from build123d import *

# Parameters (mm, degrees)
F1_DEPTH = 20
F2_R     = 30
F3_T     = -2.5
F4_W     = 2.5
F4_H     = 2.5
F5_DEPTH = 15


with BuildPart() as f1:
    # F0 (on Top) → F1 (new body)
    with BuildSketch(Plane.XY):
        Polygon((44.264942, 20), (-55.735058, 20), (-55.735058, 0), (23.424878, -7.109921), (44.264942, 0), align=None)
    extrude(amount=F1_DEPTH)

    # F2
    f2_edges = [f1.edges().sort_by_distance(p)[0] for p in [
        (23.424878, -7.109921, 10),
    ]]
    fillet(f2_edges, radius=F2_R)

    # F3
    f3_openings = [f1.faces().sort_by_distance(p)[0] for p in [
        (44.264942, 10, 10),
        (-5.735058, 20, 10),
    ]]
    offset(amount=F3_T, openings=f3_openings)

    # F4 (on face) → F5 (join)
    with BuildSketch(Plane(origin=(0, 0, 17.5), x_dir=(1, 0, 0), z_dir=(0, 0, -1))):
        with Locations((43.014942, -18.75)):
            Rectangle(F4_W, F4_H)
    extrude(amount=F5_DEPTH)


solid = f1.part
Model file for the job. Use its own axes, mm. A direction names the side the tool comes from. Give positions to 0.01 mm unless a question says otherwise; leave off trailing zeros. Order: outer loops, then holes, each group sorted by start corner. A loop starts at its lowest first (then second) coordinate and runs counter-clockwise, first axis right, second up. Notation, with made-up numbers: (52, 27) - (77, 27) arc R25 cw to (77, 48) - close; hole circle Ø7 at (0.5, -35). An arc over 180 degrees is marked (long way). Write item = value, one per line. Start each with the question number.
1. Cut at D-D, the plane z = 18.75. List the corners of the cut face in (x, y), and give its area (3 significant figures).
2. Probe line 1 along Z through (x, y) = (-46, 18.25); line 2 along X through (y, z) = (16.5, 4.5); line 3 along X through (y, z) = (18, 10). List the from-to ranges inside material, lowest first.
3. Cut at A-A, the plane z = 11.5. List the corners of the cut face in (x, y).
4. Two-plate mould, pull along Y, no slides. Class faces 1 (the flat face through (43, 17.5, 10)), 2 (the flat face through (-18.459, -0.838, 9.895)), 3 (the flat face through (36.755, -2.562, 9.86)), 4 (the flat face through (41.765, 19, 10)): pulls with the +Y half, pulls with the -Y half, needs draft (parallel to the pull), parting line crosses it, or undercut.
5. Cut at C-C, the plane y = -1. List the corners of the cut face in (x, z).
6. Drop flat-ended pins along their axis: P1, Ø2, axis at x = 43.5, z = 10, coming from the -Y side; P2, Ø2, axis at x = -8, z = 4.5, coming from the +Y side; P3, Ø6, axis at x = 0, z = 3, coming from the -Y side. Give the stop position or say it passes through.
7. Which spindle directions (+Z, -Z, +X, -X, +Y, -Y) get a long thin tool onto all of the face, cutting with end or side? Do faces 5 (the cylindrical face through (22.967, -3.974, 10.105)), 6 (the flat face through (-6, 20, 18)). Say none if no direction does.
8. Cut at B-B, the plane y = 12.25. List the corners of the cut face in (x, z).
Taken from the geometry:
q1.outline = (-55.74, 0) - (17.08, -6.54) arc R30 ccw to (29.45, -5.05) - (44.26, 0) - (44.26, 20) - (-55.74, 20) - close
q1.area = 2,350 mm²
q2.line_1 = 0 to 2.5, 17.5 to 20
q2.line_2 = -55.74 to -53.24
q2.line_3 = -55.74 to -53.24, 41.76 to 44.26
q3.outline = (-55.74, 0) - (17.08, -6.54) arc R30 ccw to (29.45, -5.05) - (44.26, 0) - (44.26, 2.64) - (28.65, -2.69) arc R27.5 cw to (17.31, -4.05) - (-53.24, 2.29) - (-53.24, 20) - (-55.74, 20) - close; (41.76, 17.5) - (44.26, 17.5) - (44.26, 20) - (41.76, 20) - close
q4.face_1 = undercut
q4.face_2 = pulls with the +Y half
q4.face_3 = pulls with the -Y half
q4.face_4 = needs draft
q5.outline = (-44.6, 0) - (41.33, 0) - (41.33, 20) - (-44.6, 20) - close; hole (-16.65, 2.5) - (33.59, 2.5) - (33.59, 17.5) - (-16.65, 17.5) - close
q6.P1 = -0.6
q6.P2 = -1.69
q6.P3 = -5.28
q7.face_5 = +Y
q7.face_6 = +Z, -Z, +X, -X, +Y
q8.outline = (-55.74, 0) - (44.26, 0) - (44.26, 2.5) - (-53.24, 2.5) - (-53.24, 17.5) - (44.26, 17.5) - (44.26, 20) - (-55.74, 20) - close
